from build123d import *

# Parameters (mm, degrees)
SKETCH2_W               = 29.4
SKETCH2_H               = 24.4
BOSS_EXTRUDE1_DEPTH     = 35
SKETCH4_W               = 71
SKETCH4_H               = 24.4
BOSS_EXTRUDE2_DEPTH     = 5
SKETCH5_W               = 5
SKETCH5_H               = 100
BOSS_EXTRUDE3_DEPTH     = 24.4
BOSS_EXTRUDE5_DEPTH     = 24.4
CUT_EXTRUDE1_DEPTH      = 116.054406213
CUT_EXTRUDE1_DEPTH_BACK = 116.054406213
SKETCH3_W               = 24.4
SKETCH3_H               = 19.4


with BuildPart() as part:
    # Sketch2 → Boss-Extrude1 (new body)
    with BuildSketch(Plane(origin=(0, 0, 0), x_dir=(1, 0, 0), z_dir=(0, 1, 0))):
        Rectangle(SKETCH2_W, SKETCH2_H)
    extrude(amount=BOSS_EXTRUDE1_DEPTH)

    # Sketch4 → Boss-Extrude2 (add)
    with BuildSketch(Plane(origin=(0, 35, 0), x_dir=(1, 0, 0), z_dir=(0, 1, 0))):
        with Locations((-20.8, 0)):
            Rectangle(SKETCH4_W, SKETCH4_H)
    extrude(amount=BOSS_EXTRUDE2_DEPTH)

    # Sketch5 → Boss-Extrude3 (add)
    with BuildSketch(Plane.XY.offset(12.2)):
        with Locations((-53.8, -15)):
            Rectangle(SKETCH5_W, SKETCH5_H)
    extrude(amount=-BOSS_EXTRUDE3_DEPTH)

    # Sketch7 → Boss-Extrude5 (add)
    with BuildSketch(Plane.XY.offset(12.2)):
        with BuildLine():
            Line((-51.3, -65), (-56.3, -65))
            ThreePointArc((-56.3, -65), (-66.925596508, -75.625596508), (-77.551193015, -65))
            Line((-77.551193015, -65), (-81.625038444, -65))
            ThreePointArc((-81.625038444, -65), (-66.462519222, -80.162519222), (-51.3, -65))
        make_face()
        with BuildLine():
            Line((-81.625038444, 35), (-77.551193015, 35))
            ThreePointArc((-77.551193015, 35), (-66.925596508, 24.374403492), (-56.3, 35))
            Line((-56.3, 35), (-51.3, 35))
            ThreePointArc((-51.3, 35), (-66.462519222, 19.837480778), (-81.625038444, 35))
        make_face()
    extrude(amount=-BOSS_EXTRUDE5_DEPTH)

    # Sketch3 → Cut-Extrude1 (cut, two sides: drawn at the far end of the back side and taken through both)
    with BuildSketch(Plane.XZ.offset(-CUT_EXTRUDE1_DEPTH_BACK)):
        Rectangle(SKETCH3_W, SKETCH3_H)
    extrude(amount=CUT_EXTRUDE1_DEPTH + CUT_EXTRUDE1_DEPTH_BACK, mode=Mode.SUBTRACT)


solid = part.part
Part model, mm, in its own coordinate system. A direction names the side the tool comes from. Round coordinates to 2 decimals unless told otherwise and drop trailing zeros. Write each loop counter-clockwise with the first axis right and the second up, starting at its lowest first coordinate (ties: lowest second). Pieces come first, ordered by that corner, then holes. Notation, with made-up numbers: M 85,52 L 113,52 A7 cw 113,63 Z; hole C -30.5,11.5 d7. An arc over 180 degrees is marked long. Return JSON: item names as keys, results as strings. Group by question number.
(1) Saw through at B-B on y = 29. Write the cut outline in (x, z).
(2) Which spindle directions (+Z, -Z, +X, -X, +Y, -Y) get a long thin tool onto all of the face, cutting with end or side? Do faces 1 (the face through (-66.692, -75.623, 0.171)), 2 (the face through (-51.3, -16, 0)), 3 (the face through (-80, 35, 0)). Say none if no direction does.
(3) Two-plate mould, pull along Y, no slides. Class faces 4 (the face through (-56.3, -21, 0)), 5 (the face through (-33, 35, 0)), 6 (the face through (0, 20, 9.7)): +Y half, -Y half, draft (parallel to the pull), parting line (faces both ways), or undercut.
(4) Pin check, flat tips, straight feed: pin 1 Ø3 at (y, z) = (-49.5, 7.5) entering from +X; pin 2 Ø3.5 at (x, z) = (-79.5, 3) entering from +Y; pin 3 Ø2.5 at (y, z) = (36.5, -5) entering from -X. Stop position of each tip, or through.
(5) Saw through at C-C on x = -38. Write the cut outline in (y, z), then the cut area to 3 significant figures.
(6) Drill centre lines: probe 1 along X at (y, z) = (1, -1.25); probe 2 along X at (y, z) = (25.5, -8.75); probe 3 along X at (y, z) = (30, -0.25). Where is each one in solid material? Low to high.
(7) Saw through at D-D on y = -34. Write the cut outline in (x, z), then the cut area to 3 significant figures.
Returned:
{
 "1": {"outline": "M -80.39,-12.2 L -75.7,-12.2 L -75.7,12.2 L -80.39,12.2 Z; M -58.16,-12.2 L -51.3,-12.2 L -51.3,12.2 L -58.16,12.2 Z; M -14.7,-12.2 L 14.7,-12.2 L 14.7,12.2 L -14.7,12.2 Z; hole M -12.2,-9.7 L 12.2,-9.7 L 12.2,9.7 L -12.2,9.7 Z"},
 "2": {"face 1": "+Z, -Z", "face 2": "+Z, -Z, -Y", "face 3": "+Z, -Z, -X, +Y"},
 "3": {"face 4": "undercut", "face 5": "-Y half", "face 6": "draft"},
 "4": {"pin 1": "x = -51.3", "pin 2": "y = 35", "pin 3": "x = -56.3"},
 "5": {"outline": "M 35,-12.2 L 40,-12.2 L 40,12.2 L 35,12.2 Z", "area": "122 mm²"},
 "6": {"probe 1": "-56.3 to -51.3, -14.7 to -12.2, 12.2 to 14.7", "probe 2": "-78.28 to -71.69, -62.17 to -51.3, -14.7 to -12.2, 12.2 to 14.7", "probe 3": "-80.78 to -76.3, -57.55 to -51.3, -14.7 to -12.2, 12.2 to 14.7"},
 "7": {"outline": "M -56.3,-12.2 L -51.3,-12.2 L -51.3,12.2 L -56.3,12.2 Z", "area": "122 mm²"}
}
